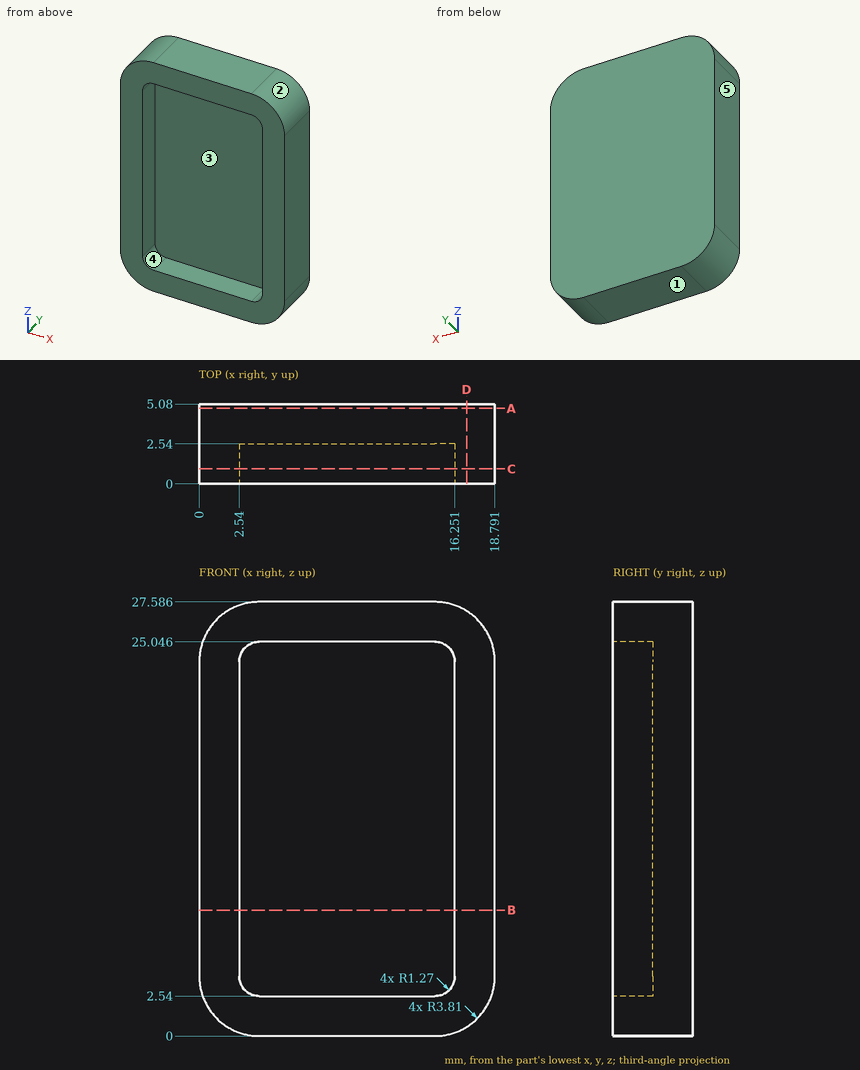
Can you work these out from the drawing? Everything is in mm from the part's minimum corner. A direction names the side the tool comes from. Coordinates: 2 decimals unless noted, no trailing zeros. Loops run counter-clockwise (first coordinate to the right, second up) from the corner with the lowest first, then second, coordinate; pieces in that order, holes last.
1) Imagine slicing it at C-C on y = 0.95. List the corners of the cut face in (x, z) for me.
2) For pin 1 (7 mm diameter, centred on x = 11.5, z = 18.5, fed in from -Y), with a flat end and sliding along its axis, tell me the tip position at first contact or that it passes through.
3) Imagine slicing it at D-D on x = 17. List the corners of the cut face in (y, z) for me, plus the area to 3 significant figures.
4) I need wall thicknesses on probe 1 along X at (y, z) = (1.85, 17.5); probe 2 along Z at (x, y) = (11, 0.7); probe 3 along Y at (x, z) = (12, 7.5). Which ranges of each line are inside material? Lowest first, please.
5) Imagine slicing it at B-B on z = 8. List the corners of the cut face in (x, y) for me.
6) Which directions (+Z, -Z, +X, -X, +Y, -Y) give clear straight access to the entire face, cutting with the end or side of a thin tool? Please do the marked faces 4 and 5.
7) Imagine slicing it at A-A on y = 4.8. List the corners of the cut face in (x, z) for me.
8) Thinking about a two-plate mould opening in Z: for the marked faces 1, 2 and 3, which applies, pulls with the +Z half, pulls with the -Z half, needs draft (parallel to the pull), parting line crosses it, or undercut?
Completed:
1. outline: (0, 3.81) arc R3.81 ccw to (3.81, 0) - (14.98, 0) arc R3.81 ccw to (18.79, 3.81) - (18.79, 23.78) arc R3.81 ccw to (14.98, 27.59) - (3.81, 27.59) arc R3.81 ccw to (0, 23.78) - close; hole (2.54, 3.81) arc R1.27 ccw to (3.81, 2.54) - (14.98, 2.54) arc R1.27 ccw to (16.25, 3.81) - (16.25, 23.78) arc R1.27 ccw to (14.98, 25.05) - (3.81, 25.05) arc R1.27 ccw to (2.54, 23.78) - close
2. pin 1: stops at y = 2.54
3. outline: (0, 0.58) - (5.08, 0.58) - (5.08, 27.01) - (0, 27.01) - close
3. area: 134 mm2
4. probe 1: x = 0 to 2.54, 16.25 to 18.79
4. probe 2: z = 0 to 2.54, 25.05 to 27.59
4. probe 3: y = 2.54 to 5.08
5. outline: (0, 0) - (2.54, 0) - (2.54, 2.54) - (16.25, 2.54) - (16.25, 0) - (18.79, 0) - (18.79, 5.08) - (0, 5.08) - close
6. face 4: -Y
6. face 5: +Z, -Z, -X, +Y, -Y
7. outline: (0, 3.81) arc R3.81 ccw to (3.81, 0) - (14.98, 0) arc R3.81 ccw to (18.79, 3.81) - (18.79, 23.78) arc R3.81 ccw to (14.98, 27.59) - (3.81, 27.59) arc R3.81 ccw to (0, 23.78) - close
8. face 1: pulls with the -Z half
8. face 2: pulls with the +Z half
8. face 3: undercut
